Here's the drawing with two shaded views (mm, measured from the low corner). I have some questions. A direction names the side the tool comes from. Round coordinates to 2 decimals unless told otherwise and drop trailing zeros. Order: outer loops, then holes, each group sorted by start corner. A loop starts at its lowest first (then second) coordinate and runs counter-clockwise, first axis right, second up. Notation, with made-up numbers: (44.5, 38) -> (72.5, 38) arc R30 ccw to (72.5, 76) -> close; hole circle Ø10 at (18.25, -20.5). An arc over 180 degrees is marked (long way). Answer in a Markdown table with one row per item.
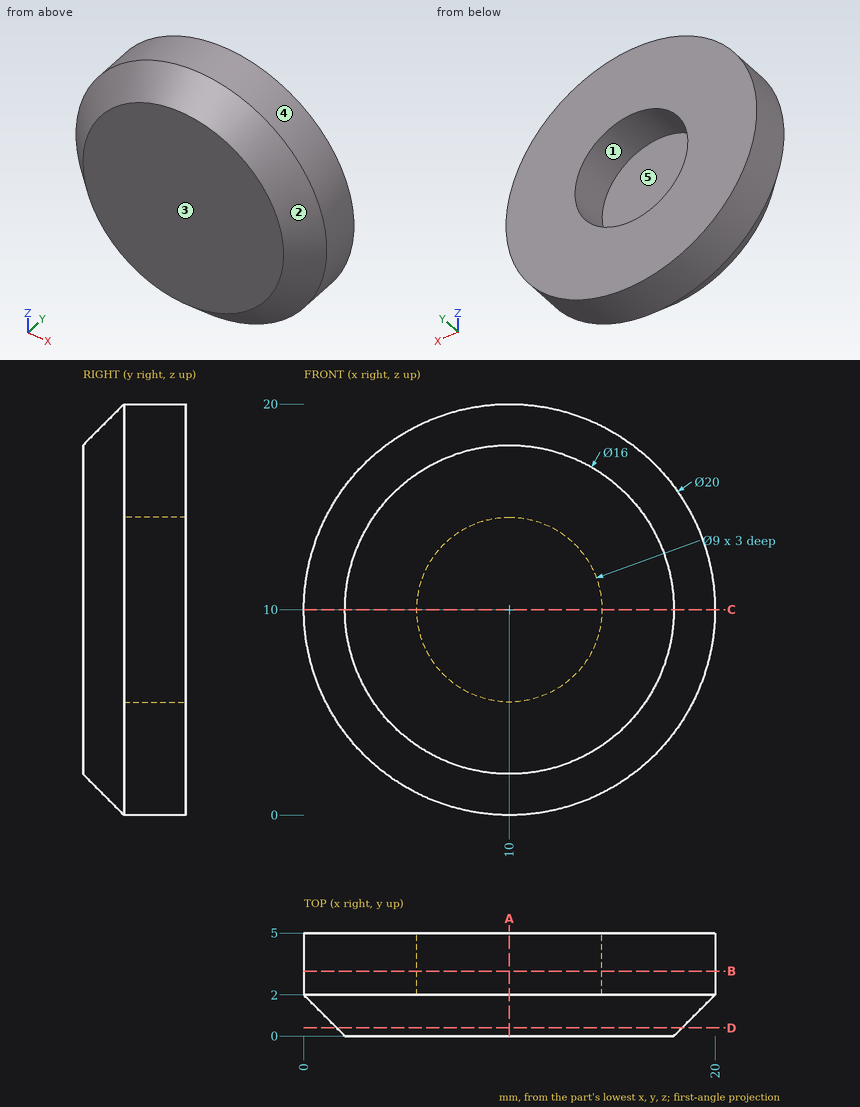
1. For pin 1 Ø3 at (x, y) = (6.5, 4) entering from +Z; pin 2 Ø4.5 at (x, z) = (9.5, 8.5) entering from +Y, each with a flat end and sliding along its axis, tell me the tip position at first contact or that it passes through.
Numbers:
| item | result |
|---|---|
| pin 1 | stops at z = 19.8 |
| pin 2 | stops at y = 2 |
2. Please list where these lines run through material, in increasing order: line 1 along X through (y, z) = (4.3, 10); line 2 along Y through (x, z) = (10, 6.5); line 3 along Z through (x, y) = (9, 4.6).
Numbers:
| item | result |
|---|---|
| line 1 | x = 0 to 5.5, 14.5 to 20 |
| line 2 | y = 0 to 2 |
| line 3 | z = 0.05 to 5.61, 14.39 to 19.95 |
3. Suppose I cut it at D-D on y = 0.4. Write out the boundary of the cut face in (x, z).
Numbers:
| item | result |
|---|---|
| outline | circle Ø16.8 at (10, 10) |
4. We'd pull the mould along X, two halves only. Please class the marked faces 3, 4 and 5: released by +X, released by -X, zero draft, split by the parting line, or undercut.
Numbers:
| item | result |
|---|---|
| face 3 | zero draft |
| face 4 | split by the parting line |
| face 5 | undercut |
5. Suppose I cut it at A-A on x = 10. Write out the boundary of the cut face in (y, z).
Numbers:
| item | result |
|---|---|
| outline | (0, 2) -> (2, 0) -> (5, 0) -> (5, 5.5) -> (2, 5.5) -> (2, 14.5) -> (5, 14.5) -> (5, 20) -> (2, 20) -> (0, 18) -> close |
6. Suppose I cut it at C-C on z = 10. Write out the boundary of the cut face in (x, y), then the cut area to 3 significant figures.
Numbers:
| item | result |
|---|---|
| outline | (0, 2) -> (2, 0) -> (18, 0) -> (20, 2) -> (20, 5) -> (14.5, 5) -> (14.5, 2) -> (5.5, 2) -> (5.5, 5) -> (0, 5) -> close |
| area | 69.0 mm2 |
7. Suppose I cut it at B-B on y = 3.15. Write out the boundary of the cut face in (x, z), then the cut area to 3 significant figures.
Numbers:
| item | result |
|---|---|
| outline | circle Ø20 at (10, 10); hole circle Ø9 at (10, 10) |
| area | 251 mm2 |
8. For the marked faces 1 and 2, which set-ups out of +Z, -Z, +X, -X, +Y, -Y let a thin tool reach every point of the face, with its end or its side?
Numbers:
| item | result |
|---|---|
| face 1 | +Y |
| face 2 | -Y |
